Work out the finished part from the listing and answer in its coordinate system (mm). A direction names the side the tool comes from. Coordinates: 2 decimals unless noted, no trailing zeros. Write each loop counter-clockwise with the first axis right and the second up, starting at its lowest first coordinate (ties: lowest second). Pieces come first, ordered by that corner, then holes. Notation, with made-up numbers: (-24.5, -1.75) - (8.5, -1.75) arc R14 cw to (8.5, 25.25) - close; hole circle Ø9 at (-0.5, 85.25). An arc over 180 degrees is marked (long way). Use CSV: the item, a comma, the result in double quotes. Start each with the question number.
from build123d import *

# Parameters (mm, degrees)
BOSS_EXTRUDE1_DEPTH = 6.35
SKETCH2_R           = 2.921
CUT_EXTRUDE1_DEPTH  = 92.800885072
FILLET1_R           = 12.7


with BuildPart() as part:
    # Sketch1 → Boss-Extrude1 (new body)
    with BuildSketch(Plane.XY):
        Polygon((0, 0), (0, 50.8), (25.4, 50.8), (25.4, 25.4), (76.2, 25.4), (76.2, 0), align=None)
    extrude(amount=BOSS_EXTRUDE1_DEPTH)

    # Sketch2 → Cut-Extrude1 (cut, through all)
    with BuildSketch(Plane.XY.offset(6.35)):
        with Locations((12.7, 38.1)):
            Circle(SKETCH2_R)
        with Locations((12.7, 12.7)):
            Circle(SKETCH2_R)
        with Locations((38.1, 12.7)):
            Circle(SKETCH2_R)
        with Locations((63.5, 12.7)):
            Circle(SKETCH2_R)
    extrude(amount=-CUT_EXTRUDE1_DEPTH, mode=Mode.SUBTRACT)

    # Fillet1
    fillet1_edges = [part.edges().sort_by_distance(p)[0] for p in [
        (25.4, 25.4, 3.175),
    ]]
    fillet(fillet1_edges, radius=FILLET1_R)


solid = part.part
Item 1: Which of the six approach directions +Z, -Z, +X, -X, +Y, -Y give full straight-line access (tool end or side, diameter ignored) to faces 4 (the face through (57, 25.4, 3)), 5 (the face through (60.58, 12.83, 3.22))?
Item 2: Each of these flat-tipped pins is pushed along its axis until it touches: pin 1 (3 mm diameter, centred on x = 62, z = 4.5, fed in from +Y); pin 2 (2 mm diameter, centred on x = 32, z = 4.5, fed in from +Y). Where does it stop, or does it pass through?
Item 3: A cutting plane is placed at D-D (x = 63.5). Determine the outline of the cut face in (y, z).
Item 4: Determine the mould class of faces 1 (the face through (39, 0, 3)), 2 (the face through (25.4, 45, 3)), 3 (the face through (40.798, 11.581, 3.219)) for opening direction X: +X half, -X half, draft (parallel to the pull), parting line (faces both ways), or undercut.
Item 5: A cutting plane is placed at B-B (x = 12.7). Determine the outline of the cut face in (y, z).
Item 6: A cutting plane is placed at A-A (z = 4). Determine the outline of the cut face in (x, y).
Item 7: A cutting plane is placed at C-C (x = 39.5). Determine the outline of the cut face in (y, z), then the cut area to 3 significant figures.
Item 8: Straight lines are drawn through the part: probe 1 along Y at (x, z) = (12.7, 3); probe 2 along X at (y, z) = (13.5, 1); probe 3 along Y at (x, z) = (12, 0.75). For each, find the intervals that lie inside material, in ascending order. Write a range as [from, to].
Calculated:
1,face 4,"+Z, -Z, +X, +Y"
1,face 5,"+Z, -Z"
2,pin 1,"stops at y = 25.4"
2,pin 2,"stops at y = 27.57"
3,outline,"(0, 0) - (9.78, 0) - (9.78, 6.35) - (0, 6.35) - close; (15.62, 0) - (25.4, 0) - (25.4, 6.35) - (15.62, 6.35) - close"
4,face 1,"draft"
4,face 2,"+X half"
4,face 3,"undercut"
5,outline,"(0, 0) - (9.78, 0) - (9.78, 6.35) - (0, 6.35) - close; (15.62, 0) - (35.18, 0) - (35.18, 6.35) - (15.62, 6.35) - close; (41.02, 0) - (50.8, 0) - (50.8, 6.35) - (41.02, 6.35) - close"
6,outline,"(0, 0) - (76.2, 0) - (76.2, 25.4) - (38.1, 25.4) arc R12.7 cw to (25.4, 38.1) - (25.4, 50.8) - (0, 50.8) - close; hole circle Ø5.84 at (12.7, 12.7); hole circle Ø5.84 at (12.7, 38.1); hole circle Ø5.84 at (38.1, 12.7); hole circle Ø5.84 at (63.5, 12.7)"
7,outline,"(0, 0) - (10.14, 0) - (10.14, 6.35) - (0, 6.35) - close; (15.26, 0) - (25.4, 0) - (25.4, 6.35) - (15.26, 6.35) - close"
7,area,"129 mm²"
8,probe 1,"y = [0, 9.78], [15.62, 35.18], [41.02, 50.8]"
8,probe 2,"x = [0, 9.89], [15.51, 35.29], [40.91, 60.69], [66.31, 76.2]"
8,probe 3,"y = [0, 9.86], [15.54, 35.26], [40.94, 50.8]"
